Drawing for the job (mm, zero at the part's lowest x, y, z). A direction names the side the tool comes from. Round coordinates to 2 decimals unless told otherwise and drop trailing zeros. Write each loop counter-clockwise with the first axis right and the second up, starting at its lowest first coordinate (ties: lowest second). Pieces come first, ordered by that corner, then holes. Notation, with made-up numbers: (25.25, -26) - (54.25, -26) arc R10 ccw to (54.25, -20) - close; hole circle Ø1 at (-8, 37.5). An arc over 180 degrees is marked (long way). One line per question, with ' | ' between items.
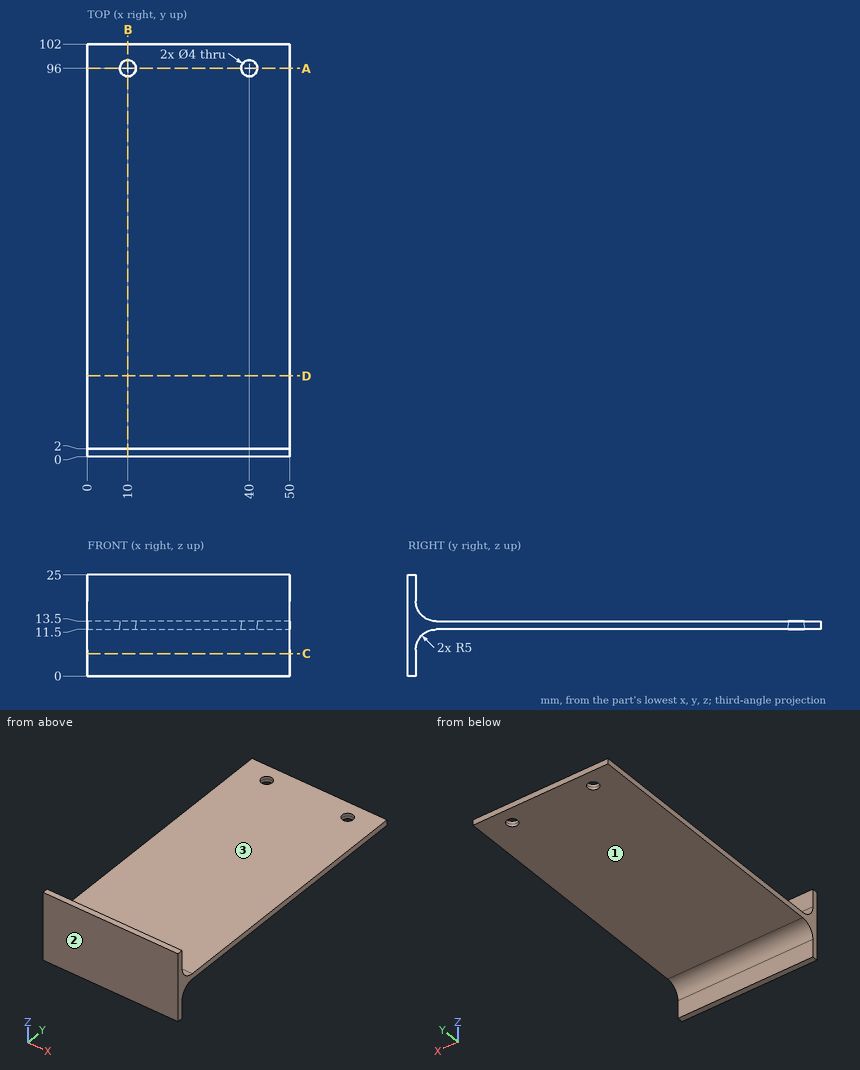
Q1. Saw through at A-A, the plane y = 96. List the corners of the cut face in (x, z), then the cut area to 3 significant figures.
Found:
outline: (0, 11.5) - (8, 11.5) - (8, 13.5) - (0, 13.5) - close; (12, 11.5) - (38, 11.5) - (38, 13.5) - (12, 13.5) - close; (42, 11.5) - (50, 11.5) - (50, 13.5) - (42, 13.5) - close | area: 84.0 mm^2
Q2. Drop flat-ended pins along their axis: pin 1 (1.5 mm diameter, centred on x = 30, z = 6, fed in from -Y); pin 2 (4.5 mm diameter, centred on x = 10, y = 96, fed in from -Z); pin 3 (3.5 mm diameter, centred on x = 10, y = 96, fed in from -Z); pin 4 (3.5 mm diameter, centred on x = 26, z = 20.5, fed in from +Y). Give the stop position or say it passes through.
Found:
pin 1: y = 0 | pin 2: z = 11.5 | pin 3: through | pin 4: y = 2
Q3. Drill centre lines: L1, parallel to X at y = 96, z = 13.1; L2, parallel to Y at x = 40, z = 12.8; L3, parallel to Z at x = 14.5, y = 41. Where is each one in solid material? Low to high. Write a range as from..to.
Found:
L1: 0..8, 12..38, 42..50 | L2: 0..94, 98..102 | L3: 11.5..13.5
Q4. Saw through at C-C, the plane z = 5.5. List the corners of the cut face in (x, y), then the cut area to 4 significant figures.
Found:
outline: (0, 0) - (50, 0) - (50, 2) - (0, 2) - close | area: 100.0 mm^2
Q5. Saw through at D-D, the plane y = 20. List the corners of the cut face in (x, z).
Found:
outline: (0, 11.5) - (50, 11.5) - (50, 13.5) - (0, 13.5) - close
Q6. Saw through at B-B, the plane x = 10. List the corners of the cut face in (y, z).
Found:
outline: (0, 0) - (2, 0) - (2, 6.5) arc R5 cw to (7, 11.5) - (94, 11.5) - (94, 13.5) - (7, 13.5) arc R5 cw to (2, 18.5) - (2, 25) - (0, 25) - close; (98, 11.5) - (102, 11.5) - (102, 13.5) - (98, 13.5) - close
Q7. Which spindle directions (+Z, -Z, +X, -X, +Y, -Y) get a long thin tool onto all of the face, cutting with end or side? Do the marked faces 1, 2 and 3. Say none if no direction does.
Found:
face 1: -Z, +X, -X, +Y | face 2: +Z, -Z, +X, -X, -Y | face 3: +Z, +X, -X, +Y
